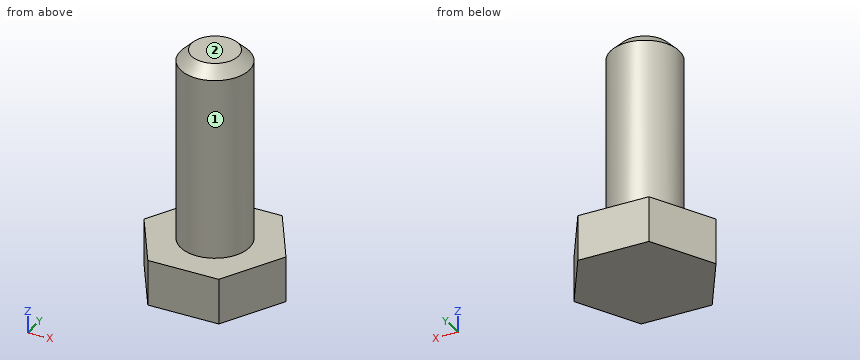
```python
from build123d import *

# Parameters (mm, degrees)
DODANIE_WYCI_GNI_CIE1_DEPTH = 4.15
SZKIC2_R                    = 3.11
DODANIE_WYCI_GNI_CIE2_DEPTH = 17.5
SFAZOWANIE1_SIZE            = 1


with BuildPart() as part:
    # Szkic1 → Dodanie-wyciągnięcie1 (new body)
    with BuildSketch(Plane.XY):
        Polygon((-3.229086971, 5.468668089), (-6.350548975, -0.062137304), (-3.121462004, -5.530805393), (3.229086971, -5.468668089), (6.350548975, 0.062137304), (3.121462004, 5.530805393), align=None)
    extrude(amount=DODANIE_WYCI_GNI_CIE1_DEPTH)

    # Szkic2 → Dodanie-wyciągnięcie2 (add)
    with BuildSketch(Plane.XY.offset(4.15)):
        Circle(SZKIC2_R)
    extrude(amount=DODANIE_WYCI_GNI_CIE2_DEPTH)

    # Sfazowanie1
    sfazowanie1_edges = [part.edges().sort_by_distance(p)[0] for p in [
        (-3.11, 0, 21.65),
    ]]
    chamfer(sfazowanie1_edges, length=SFAZOWANIE1_SIZE)


solid = part.part
```
Geometry check sheet. Reference: the model listing, model coordinates, mm. Face numbers are marked on the shaded views. A direction names the side the tool comes from. Coordinates: 2 decimals unless noted, no trailing zeros. Write each loop counter-clockwise with the first axis right and the second up, starting at its lowest first coordinate (ties: lowest second). Pieces come first, ordered by that corner, then holes. Notation, with made-up numbers: (83.5, 3.5) -> (126.5, 3.5) arc R19 cw to (126.5, 13.5) -> close; hole circle Ø2 at (25.5, 5). An arc over 180 degrees is marked (long way). Use CSV: the item, a comma, the result in double quotes. Start each with the question number.
Item 1: Cross-section at C-C, the plane z = 8. Record the cut outline in (x, y), plus the area to 3 significant figures.
Item 2: Cross-section at D-D, the plane x = 4. Record the cut outline in (y, z).
Item 3: Set-up check for the marked faces 1 and 2: record each of +Z, -Z, +X, -X, +Y, -Y from which the full face is reachable in a straight line by a thin tool's end or side.
Item 4: Cross-section at B-B, the plane x = 0. Record the cut outline in (y, z).
Item 5: Thickness scan on line 1 (Z direction, x = -4, y = 4); line 2 (Y direction, x = -1.5, z = 3.25); line 3 (X direction, y = -1.5, z = 8.25). Record the ranges inside material, lowest first.
Item 6: Cross-section at A-A, the plane z = 3.25. Record the cut outline in (x, y), plus the area to 3 significant figures.
Item 7: Depth check by flat-ended pin: pin 1 Ø1 at (x, z) = (-1, 5) entering from +Y; pin 2 Ø1.5 at (x, z) = (-0.5, 13) entering from -Y; pin 3 Ø6 at (x, z) = (-4.5, 15) entering from -Y. Enter the tip coordinate at first touch or a pass-through.
Answers:
1,outline,"circle Ø6.22 at (0, 0)"
1,area,"30.4 mm^2"
2,outline,"(-4.1, 0) -> (4.04, 0) -> (4.04, 4.15) -> (-4.1, 4.15) -> close"
3,face 1,"+Z"
3,face 2,"+Z, +X, -X, +Y, -Y"
4,outline,"(-5.5, 0) -> (5.5, 0) -> (5.5, 4.15) -> (3.11, 4.15) -> (3.11, 20.65) -> (2.11, 21.65) -> (-2.11, 21.65) -> (-3.11, 20.65) -> (-3.11, 4.15) -> (-5.5, 4.15) -> close"
5,line 1,"0 to 4.15"
5,line 2,"-5.51 to 5.49"
5,line 3,"-2.72 to 2.72"
6,outline,"(-6.35, -0.06) -> (-3.12, -5.53) -> (3.23, -5.47) -> (6.35, 0.06) -> (3.12, 5.53) -> (-3.23, 5.47) -> close"
6,area,"105 mm^2"
7,pin 1,"y = 3.07"
7,pin 2,"y = -3.11"
7,pin 3,"y = -2.72"
